Check sheet for the modelled part. Datum: model origin and axes. Units: mm. Face numbers are marked on the shaded views. A direction names the side the tool comes from. Give positions to 0.01 mm unless a question says otherwise; leave off trailing zeros. Write each loop counter-clockwise with the first axis right and the second up, starting at its lowest first coordinate (ties: lowest second). Pieces come first, ordered by that corner, then holes. Notation, with made-up numbers: M 37,3 L 81,3 A24 ccw 81,23 Z; hole C 41,59 d4. An arc over 180 degrees is marked long. One line per item, written item: value. Start each with the question number.
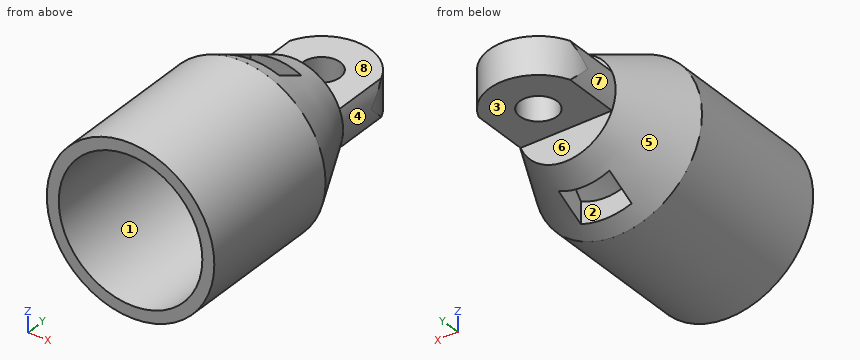
from build123d import *

# Parameters (mm, degrees)
SKETCH1_R           = 7.112
SKETCH1_R_2         = 6.096
BOSS_EXTRUDE1_DEPTH = 12.7
SKETCH3_R           = 1.5875
BOSS_EXTRUDE3_DEPTH = 1.5875
CUT_EXTRUDE1_DEPTH  = 12.7
SKETCH5_OUTSIDE_W   = 22.798
SKETCH5_OUTSIDE_H   = 22.798
SKETCH5_OUTSIDE_R   = 4.191
CUT_EXTRUDE3_DEPTH  = 25.4


with BuildPart() as part:
    # Sketch1 → Boss-Extrude1 (new body)
    with BuildSketch(Plane(origin=(0, 0, 0), x_dir=(1, 0, 0), z_dir=(0, 1, 0))):
        Circle(SKETCH1_R)
        Circle(SKETCH1_R_2, mode=Mode.SUBTRACT)
    extrude(amount=BOSS_EXTRUDE1_DEPTH)

    # Sketch2 → Revolve2 (revolve)
    with BuildSketch(Plane.XY):
        Polygon((-7.112, 12.7), (-6.096, 12.7), (-2.159, 16.601959342), (0, 16.601959342), (0, 18.633959342), (-4.191, 18.633959342), align=None)
    revolve(axis=Axis((0, 16.601959342, 0), (0, 1, 0)))

    # Sketch3 → Boss-Extrude3 (add, symmetric)
    with BuildSketch(Plane.XY):
        with BuildLine():
            Line((-4.191, 18.633959342), (-4.191, 21.808959342))
            ThreePointArc((-4.191, 21.808959342), (0, 25.999959342), (4.191, 21.808959342))
            Line((4.191, 21.808959342), (4.191, 18.633959342))
            Line((4.191, 18.633959342), (-4.191, 18.633959342))
        make_face()
        with Locations((0, 21.808959342)):
            Circle(SKETCH3_R, mode=Mode.SUBTRACT)
    extrude(amount=BOSS_EXTRUDE3_DEPTH, both=True)

    # Sketch4 → Cut-Extrude1 (cut, symmetric)
    with BuildSketch(Plane.XY):
        Polygon((0, 16.601959342), (2.159, 16.601959342), (2.159, 14.061959342), (-2.159, 14.061959342), (-2.159, 16.601959342), align=None)
    extrude(amount=CUT_EXTRUDE1_DEPTH, both=True, mode=Mode.SUBTRACT)

    # Sketch5 outside → Cut-Extrude3 (cut)
    with BuildSketch(Plane.XZ.offset(-18.633959342)):
        Rectangle(SKETCH5_OUTSIDE_W, SKETCH5_OUTSIDE_H)
        Circle(SKETCH5_OUTSIDE_R, mode=Mode.SUBTRACT)
    extrude(amount=-CUT_EXTRUDE3_DEPTH, mode=Mode.SUBTRACT)


solid = part.part
1) Cross-section at A-A (x = 0). Record the boundary of the cut face in (y, z).
2) Cross-section at C-C (y = 24). Record the boundary of the cut face in (x, z), plus the area to 3 significant figures.
3) Tool access check on the marked faces 5, 6, 7 and 8. Record the directions out of +Z, -Z, +X, -X, +Y, -Y that give a thin tool (end or side, any length) a straight path to the whole face; none if there is none.
4) Draft check along X on the marked faces 1, 2, 3 and 4. Enter one of: released by +X, released by -X, zero draft, split by the parting line, or undercut.
5) Cross-section at D-D (y = 13.75). Record the boundary of the cut face in (x, z), plus the area to 3 significant figures.
6) Material ranges on L1, parallel to X at y = 6.25, z = 0; L2, parallel to Y at x = 0, z = -0.7, recorded low to high. Write a range as from..to.
7) Gauge pin test, flat ends, axial feed: pin 1 (1.9 mm diameter, centred on x = 0, y = 21.81, fed in from +Z); pin 2 (0.8 mm diameter, centred on x = 1, z = -3.5, fed in from +Y); pin 3 (3 mm diameter, centred on y = 5, z = 2.5, fed in from +X); pin 4 (1.3 mm diameter, centred on y = 15.5, z = -1.5, fed in from -X). Record the tip position at first contact, or that the pin passes through.
8) Cross-section at B-B (y = 9). Record the boundary of the cut face in (x, z), plus the area to 3 significant figures.
Data:
1. outline: M 0,-7.11 L 12.7,-7.11 L 14.06,-6.44 L 14.06,-4.72 L 12.7,-6.1 L 0,-6.1 Z; M 0,6.1 L 12.7,6.1 L 14.06,4.72 L 14.06,6.44 L 12.7,7.11 L 0,7.11 Z; M 16.6,-5.19 L 18.63,-4.19 L 18.63,-1.59 L 20.22,-1.59 L 20.22,1.59 L 18.63,1.59 L 18.63,4.19 L 16.6,5.19 Z; M 23.4,-1.59 L 26,-1.59 L 26,1.59 L 23.4,1.59 Z
2. outline: M -3.57,-1.59 L 3.57,-1.59 L 3.57,1.59 L -3.57,1.59 Z
2. area: 22.7 mm2
3. face 5: +Y
3. face 6: -Z, +X, -X, +Y
3. face 7: -X, +Y
3. face 8: +Z, +X, -X, +Y
4. face 1: undercut
4. face 2: undercut
4. face 3: zero draft
4. face 4: released by +X
5. outline: C 0,0 d13.19; hole C 0,0 d10.07
5. area: 57.0 mm2
6. L1: x = -7.11..-6.1, 6.1..7.11
6. L2: y = 16.6..20.22, 23.4..26
7. pin 1: passes through
7. pin 2: stops at y = 18.63
7. pin 3: stops at x = 7.04
7. pin 4: stops at x = -5.9
8. outline: C 0,0 d14.22; hole C 0,0 d12.19
8. area: 42.2 mm2
